```python
from build123d import *

# Parameters (mm, degrees)
F4_DEPTH = 0.6
F5_COUNT = 3


with BuildPart() as f2:
    # F1 (on Front) → F2 (revolve)
    with BuildSketch(Plane.XZ):
        with BuildLine():
            ThreePointArc((12.049969539, 40.0034904813), (11.9095920603, 39.9424526163), (11.8534904813, 39.800030461))
            Line((11.8534904813, 39.800030461), (12.5482025971, 0))
            Line((12.5482025971, 0), (13.7480198313, 0.0209428877))
            Line((13.7480198313, 0.0209428877), (13.0533077155, 39.8209733487))
            ThreePointArc((13.0533077155, 39.8209733487), (12.9922698505, 39.9613508275), (12.8498476952, 40.0174524064))
            Line((12.8498476952, 40.0174524064), (12.049969539, 40.0034904813))
        make_face()
    revolve(axis=Axis((0, 0, 20), (0, 0, 1)))

    # F3 (on Front) → F4 (join, symmetric)
    with BuildSketch(Plane.XZ):
        Polygon((34.4769248011, 12.0279620331), (11.884605497, 38.0174524064), (12.5477969416, 0.0232399905), (44.0591547085, -35.8122301865), align=None)
    extrude(amount=F4_DEPTH, both=True)

    # F5: F2 ×3 about axis
    f5_axis = Axis((0, 0, 20), (0, 0, 1))


with BuildPart() as f2_1:
    add(f2.part)
    for i in range(1, F5_COUNT):
        add(f2.part.rotate(f5_axis, i * 360 / F5_COUNT))


solid = f2_1.part
```
Geometry: final body of the model. Coordinates: model frame, mm. A direction names the side the tool comes from. Round coordinates to 2 decimals unless told otherwise and drop trailing zeros. Order: outer loops, then holes, each group sorted by start corner. A loop starts at its lowest first (then second) coordinate and runs counter-clockwise, first axis right, second up. Notation, with made-up numbers: (13, -40) -> (45, -40) arc R24 cw to (45, -12) -> close; hole circle Ø6 at (50.25, -37.5). An arc over 180 degrees is marked (long way). Use one line per item in the form item = value. Start each with the question number.
1. Cut plane C-C (x = 26). Return the cut outline in (y, z), then the cut area to 3 significant figures.
2. Pin query (flat end, axial travel): pin 1 Ø3 at (x, y) = (11, 8) entering from -Z; pin 2 Ø15.5 at (x, z) = (34.5, 1) entering from +Y; pin 3 Ø1 at (y, z) = (-26.5, -15.5) entering from +X. Return the tip coordinate at first contact, or that it passes through.
3. Line query: probe 1 along Y at (x, z) = (-17, -20.5); probe 2 along X at (y, z) = (-10.5, 20); probe 3 along X at (y, z) = (-8, 14). Output: solid intervals per line, ascending.
4. Cut plane D-D (y = 15.5). Return the cut outline in (x, z), then the cut area to 3 significant figures.
5. Draft query along Y for faces 4 (the face through (28.093, -0.008, -17.655)), 5 (the face through (-14.05, -24.33, -17.66)), 6 (the face through (-11.975, -20.725, 24.154)), 7 (the face through (-11.961, 20.733, 24.154)). Return one class per face: pulls with the +Y half, pulls with the -Y half, needs draft (parallel to the pull), parting line crosses it, or undercut.
6. Cut plane A-A (z = 21). Return the cut outline in (x, y), then the cut area to 3 significant figures.
7. Cut plane B-B (z = -28). Return the cut outline in (x, y), then the cut area to 3 significant figures.
8. Reachability of faces 1 (the face through (-2.9, -13.08, 20.2)), 2 (the face through (-14.039, 24.333, -17.655)), 3 (the face through (11.64, 3.67, 19.62)) from +Z, -Z, +X, -X, +Y, -Y: full face, straight path, thin tool, end or side. Return the list, or none.
Solution:
q1.outline = (-0.6, -15.27) -> (0.6, -15.27) -> (0.6, 21.78) -> (-0.6, 21.78) -> close
q1.area = 44.5 mm^2
q2.pin_1 = 0
q2.pin_2 = 0.6
q2.pin_3 = -14.32
q3.probe_1 = -30.64 to -28.24, 28.24 to 30.64
q3.probe_2 = -8.32 to -6.21, 6.21 to 8.32
q3.probe_3 = -10.88 to -9.35, 9.35 to 10.88
q4.outline = (-9.64, -6.45) -> (-8.26, -5.67) -> (-8.26, 31.5) -> (-9.64, 30.7) -> close
q4.area = 51.5 mm^2
q5.face_4 = needs draft
q5.face_5 = undercut
q5.face_6 = pulls with the -Y half
q5.face_7 = pulls with the +Y half
q6.outline = (-13.86, -22.8) -> (-12.82, -23.4) -> (-6.16, -11.88) arc R13.38 ccw to (13.37, -0.6) -> (26.68, -0.6) -> (26.68, 0.6) -> (13.37, 0.6) arc R13.38 ccw to (-6.16, 11.88) -> (-12.82, 23.4) -> (-13.86, 22.8) -> (-7.2, 11.28) arc R13.38 ccw to (-7.2, -11.28) -> close; hole circle Ø24.36 at (0, 0)
q6.area = 144 mm^2
q7.outline = (-21.77, -36.5) -> (-20.73, -37.1) -> (-18.08, -32.51) -> (-19.11, -31.91) -> close; (-21.77, 36.5) -> (-19.11, 31.91) -> (-18.08, 32.51) -> (-20.73, 37.1) -> close; (37.19, -0.6) -> (42.49, -0.6) -> (42.49, 0.6) -> (37.19, 0.6) -> close
q7.area = 19.1 mm^2
q8.face_1 = +Z
q8.face_2 = -Z, +X
q8.face_3 = -Z
